For this review, take the finished solid that the model builds, in its own axes (mm). A direction names the side the tool comes from. Give positions to 0.01 mm unless a question says otherwise; leave off trailing zeros. Loops run counter-clockwise (first coordinate to the right, second up) from the corner with the lowest first, then second, coordinate; pieces in that order, holes last.
```python
from build123d import *

# Parameters (mm, degrees)
SKETCH1_R           = 1.85
SKETCH1_R_2         = 5
BOSS_EXTRUDE1_DEPTH = 4
CHAMFER1_SIZE       = 1
CUT_EXTRUDE1_DEPTH  = 166.566482115
SKETCH5_2_R         = 1.85
CUT_EXTRUDE2_DEPTH  = 4


with BuildPart() as part:
    # Sketch1 → Boss-Extrude1 (new body)
    with BuildSketch(Plane.XY):
        with BuildLine():
            Line((123.9, 7.5), (138.257864376, 7.5))
            ThreePointArc((138.257864376, 7.5), (141.59119771, 8.071909584), (144.543257987, 9.722222222))
            ThreePointArc((144.543257987, 9.722222222), (164.9, 0), (144.543257987, -9.722222222))
            ThreePointArc((144.543257987, -9.722222222), (141.59119771, -8.071909584), (138.257864376, -7.5))
            Line((138.257864376, -7.5), (123.9, -7.5))
            ThreePointArc((123.9, -7.5), (116.4, 0), (123.9, 7.5))
        make_face()
        with Locations((160.9, 0)):
            Circle(SKETCH1_R, mode=Mode.SUBTRACT)
        with Locations((152.4, 0)):
            Circle(SKETCH1_R_2, mode=Mode.SUBTRACT)
        with Locations((143.9, 0)):
            Circle(SKETCH1_R, mode=Mode.SUBTRACT)
        with Locations((133.9, 0)):
            Circle(SKETCH1_R, mode=Mode.SUBTRACT)
        with Locations((123.9, 0)):
            Circle(SKETCH1_R, mode=Mode.SUBTRACT)
    extrude(amount=BOSS_EXTRUDE1_DEPTH)

    # Chamfer1
    chamfer1_edges = [part.edges().sort_by_distance(p)[0] for p in [
        (141.59119771, 8.071909584, 4),
        (131.078932188, 7.5, 4),
        (116.4, 0, 4),
        (131.078932188, -7.5, 4),
        (141.59119771, -8.071909584, 4),
        (164.9, 0, 4),
    ]]
    chamfer(chamfer1_edges, length=CHAMFER1_SIZE)

    # Sketch3 → Revolve2 (revolve)
    with BuildSketch(Plane(origin=(152.4, 0, 0), x_dir=(0, 0, -1), z_dir=(1, 0, 0)), mode=Mode.PRIVATE) as revolve2_sk:
        Polygon((-4, -11.5), (-4, -5), (-7.671572875, -5), (-9, -3.671572875), (-9, -1.683342633), (-12, -1.683342633), (-12, -3.5), align=None)
    revolve(revolve2_sk.sketch.rotate(Axis((152.4, 0, 0), (0, 0, 1)), 270), axis=Axis((152.4, 0, 0), (0, 0, 1)))

    # Sketch4 → Cut-Extrude1 (cut, through all)
    with BuildSketch(Plane(origin=(0, 0, 4), x_dir=(-1, 0, 0), z_dir=(0, 0, -1))):
        with BuildLine():
            Line((-143.9, -3), (-141.298198344, -3))
            ThreePointArc((-141.298198344, -3), (-140.9, 0), (-141.298198344, 3))
            Line((-141.298198344, 3), (-143.9, 3))
            ThreePointArc((-143.9, 3), (-146.9, 0), (-143.9, -3))
        make_face()
    extrude(amount=-CUT_EXTRUDE1_DEPTH, mode=Mode.SUBTRACT)

    # Sketch5<2> → Cut-Extrude2 (cut)
    with BuildSketch(Plane(origin=(0, 0, 0), x_dir=(-1, 0, 0), z_dir=(0, 0, -1))):
        with Locations((-152.4, -8.5)):
            Circle(SKETCH5_2_R)
        with Locations((-152.4, 8.5)):
            Circle(SKETCH5_2_R)
    extrude(amount=-CUT_EXTRUDE2_DEPTH, mode=Mode.SUBTRACT)


solid = part.part
```
Q1. Consider section D-D on z = 7. Give the boundary of the cut face in (x, y), plus the area to 3 significant figures.
Answers:
outline: (144.43, -2.95) arc R8.5 ccw (long way) to (144.43, 2.95) arc R3 cw to start; hole circle Ø10 at (152.4, 0)
area: 135 mm2
Q2. Consider section A-A on z = 2. Give the boundary of the cut face in (x, y), plus the area to 3 significant figures.
Answers:
outline: (123.9, -7.5) - (138.26, -7.5) arc R10 cw to (144.54, -9.72) arc R12.5 ccw (long way) to (144.54, 9.72) arc R10 cw to (138.26, 7.5) - (123.9, 7.5) arc R7.5 ccw to start; hole circle Ø3.7 at (123.9, 0); hole circle Ø3.7 at (133.9, 0); hole circle Ø3.7 at (143.9, 0); hole circle Ø10 at (152.4, 0); hole circle Ø3.7 at (152.4, -8.5); hole circle Ø3.7 at (152.4, 8.5); hole circle Ø3.7 at (160.9, 0)
area: 692 mm2
Q3. Consider section B-B on x = 133.9. Give the boundary of the cut face in (y, z), plus the area to 3 significant figures.
Answers:
outline: (-7.5, 0) - (-1.85, 0) - (-1.85, 4) - (-6.5, 4) - (-7.5, 3) - close; (1.85, 0) - (7.5, 0) - (7.5, 3) - (6.5, 4) - (1.85, 4) - close
area: 44.2 mm2
Q4. For pin 1 Ø1.1 at (x, y) = (152.5, -7.5) entering from -Z; pin 2 Ø3.5 at (x, z) = (131, 1) entering from -Y; pin 3 Ø2 at (x, y) = (151.5, 1.5) entering from -Z; pin 4 Ø1.8 at (x, y) = (144, 0) entering from +Z, all flat-tipped, find the tip position at first contact; note any pin that passes through.
Answers:
pin 1: stops at z = 4
pin 2: stops at y = -7.5
pin 3: stops at z = 9
pin 4: passes through
Q5. For probe 1 along Y at (x, z) = (152.4, 2.7); probe 2 along Z at (x, y) = (149.5, -0.75); probe 3 along Y at (x, z) = (160.9, 2), list the stretches that pass through material, from the lowest coordinate up.
Answers:
probe 1: y = -12.5 to -10.35, -6.65 to -5, 5 to 6.65, 10.35 to 12.5
probe 2: z = 9 to 12
probe 3: y = -9.17 to -1.85, 1.85 to 9.17
Q6. Mouldability with a two-part tool opening along Y and no side actions: class faces 1 (the flat face through (161, 0, 4)), 2 (the cylindrical face through (164.894, 0.394, 1.479)), 3 (the flat face through (141, 0, 0)) as +Y half, -Y half, draft (parallel to the pull), parting line (faces both ways), or undercut.
Answers:
face 1: undercut
face 2: parting line
face 3: draft
Q7. Consider section C-C on z = 10.75. Give the boundary of the cut face in (x, y).
Answers:
outline: circle Ø9.5 at (152.4, 0); hole circle Ø3.37 at (152.4, 0)
Q8. Machinability: for faces 4 (the flat face through (143, -3, 5)), 5 (the flat face through (131, -7.5, 1)), 6 (the flat face through (152, -8, 4)), 7 (the flat face through (131.2, -7, 3.5)), which of the approach directions +Z, -Z, +X, -X, +Y, -Y give a long, thin tool a straight path to every point of the face, cutting with its end or side? Answer none if there is none.
Answers:
face 4: +Z, -X
face 5: +Z, -Z, -X, -Y
face 6: -Z
face 7: +Z, -X, -Y
